For this review, use the dimensioned drawing (mm, ordinates from the lowest corner) and the shaded views. Coordinates: 2 decimals unless noted, no trailing zeros. Write each loop counter-clockwise with the first axis right and the second up, starting at its lowest first coordinate (ties: lowest second). Pieces come first, ordered by that corner, then holes. Notation, with made-up numbers: (-10, 46) - (17, 46) arc R37 cw to (17, 84) - close; hole circle Ø3 at (62, -37). An arc over 180 degrees is marked (long way). One line per item, written item: value.
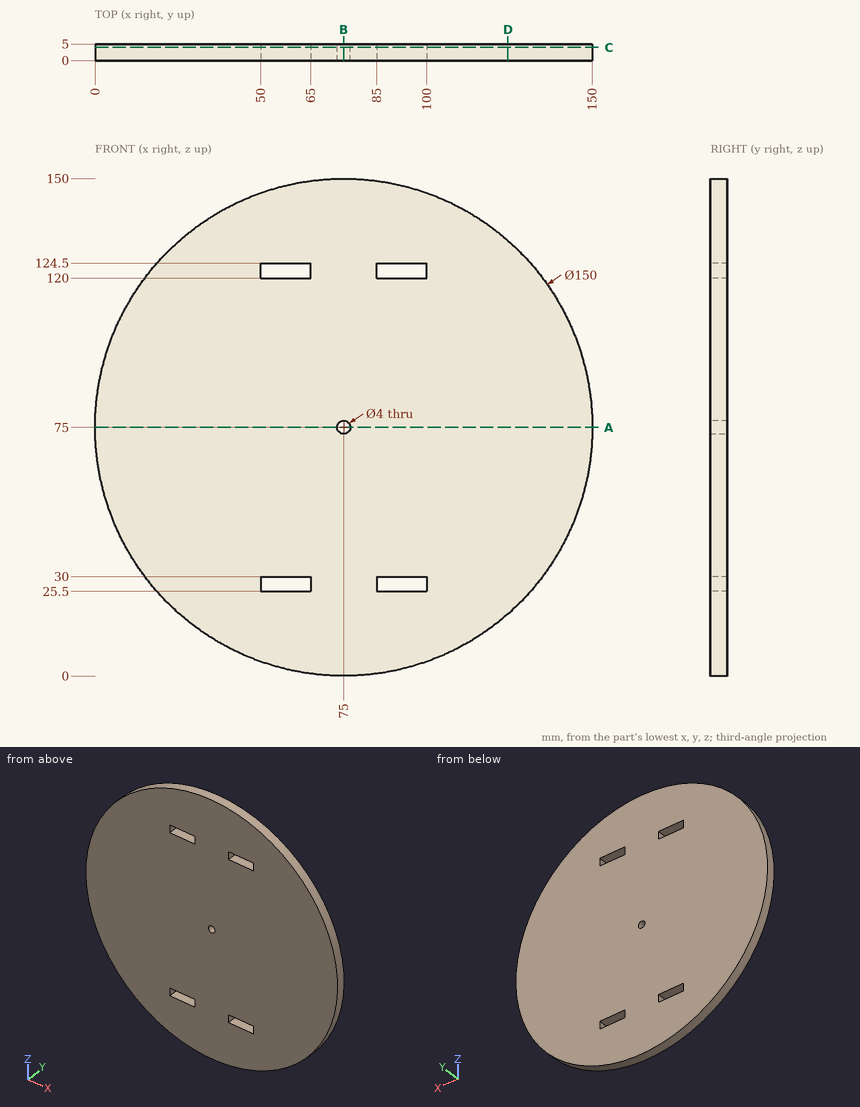
1. Consider section D-D, the plane x = 124.5. Write out the cut boundary in (y, z).
Answer block:
outline: (0, 18.66) - (5, 18.66) - (5, 131.34) - (0, 131.34) - close
2. Consider section B-B, the plane x = 75. Write out the cut boundary in (y, z).
Answer block:
outline: (0, 0) - (5, 0) - (5, 73) - (0, 73) - close; (0, 77) - (5, 77) - (5, 150) - (0, 150) - close
3. Insertion check: pin 1 Ø2.5 at (x, y) = (93.5, 3.5) entering from +Z; pin 2 Ø4.5 at (x, z) = (75, 75) entering from -Y; pin 3 Ø1.3 at (y, z) = (3, 122) entering from -X; pin 4 Ø1.5 at (x, y) = (119, 4) entering from -Z. Each pin has a flat end and moves straight along its axis. Give the tip position at first contact, or say it passes through.
Answer block:
pin 1: stops at z = 147.99
pin 2: stops at y = 0
pin 3: stops at x = 16.04
pin 4: stops at z = 13.73
4. Consider section C-C, the plane y = 4. Write out the cut boundary in (x, z).
Answer block:
outline: circle Ø150 at (75, 75); hole (50, 25.5) - (65, 25.5) - (65, 30) - (50, 30) - close; hole (50, 120) - (65, 120) - (65, 124.5) - (50, 124.5) - close; hole circle Ø4 at (75, 75); hole (85, 25.5) - (100, 25.5) - (100, 30) - (85, 30) - close; hole (85, 120) - (100, 120) - (100, 124.5) - (85, 124.5) - close
5. Wall thickness on line 1 along X through (y, z) = (1.55, 75); line 2 along Z through (x, y) = (54.5, 4.2); line 3 along X through (y, z) = (1, 17.5): over which ranges is each line inside the solid? List them lowest first.
Answer block:
line 1: x = 0 to 73, 77 to 150
line 2: z = 2.86 to 25.5, 30 to 120, 124.5 to 147.14
line 3: x = 26.85 to 123.15
6. Consider section A-A, the plane z = 75. Write out the cut boundary in (x, y), then the cut area to 3 significant figures.
Answer block:
outline: (0, 0) - (73, 0) - (73, 5) - (0, 5) - close; (77, 0) - (150, 0) - (150, 5) - (77, 5) - close
area: 730 mm^2
